Design review of the part built by this model. Coordinates are the model's own, in mm. A direction names the side the tool comes from. Coordinates: 2 decimals unless noted, no trailing zeros. Write each loop counter-clockwise with the first axis right and the second up, starting at its lowest first coordinate (ties: lowest second). Pieces come first, ordered by that corner, then holes.
Q1. The part is to be moulded in two halves that separate along Z. For faces 6 (the flat face through (-20, -57, 5)), 7 (the cylindrical face through (-15.33, -157.48, 58.78)), 8 (the conical face through (-43.789, -137.671, 58.425)), say which applies: released by +Z, released by -Z, zero draft, split by the parting line, or undercut.
Q2. Take a section at B-B, the plane z = 18.5. Write out the cut boundary in (x, y).
Q3. Take a section at A-A, the plane y = -15. Write out the cut boundary in (x, z).
Q4. For L1, parallel to Y at x = -15, z = 57; L2, parallel to Y at x = -45, z = 56.6; L3, parallel to X at y = -20, z = 48, list the stretches that pass through material, from the lowest coordinate up.
Q5. For pin 1 Ø6.5 at (x, y) = (-45, -155) entering from -Z; pin 2 Ø6 at (x, y) = (-15, -30) entering from +Z; pin 3 Ø1 at (x, z) = (-45.5, 35.5) entering from -Y, all flat-tipped, find the tip position at first contact; note any pin that passes through.
Q6. For faces 1 (the cylindrical face through (-16.75, -147.27, 2.46)), 2 (the cylindrical face through (-18.42, -162.483, 3.479)), 3 (the flat face through (-60, -79, 57)), 4 (the flat face through (-25, -160, 2)), 5 (the cylindrical face through (-42.69, -14.04, 58.78)), list the 3-axis set-ups (+Z, -Z, +X, -X, +Y, -Y) from which the entire face can be reached by the end or side of a thin tool; tool diameter is ignored.
from build123d import *

# Parameters (mm, degrees)
F0_R     = 2.5
F1_DEPTH = 5
F2_W     = 170
F2_H     = 50.3
F3_DEPTH = 5
F4_W     = 55
F4_H     = 50.3
F5_DEPTH = 5
F7_R     = 2.5
F8_DEPTH = 5
F9_SIZE  = 2
F10_SIZE = 2
F11_SIZE = 2
F12_R    = 2


# Not quite as in the source:
# - a feature names something its author has since deleted; it is built from what else it names


with BuildPart() as f1:
    # F0 (on Top) → F1 (new body)
    with BuildSketch(Plane.XY):
        with BuildLine():
            Line((-60, 0), (0, 0))
            Line((0, 0), (0, 150))
            Line((0, 150), (0, 170))
            Line((0, 170), (-15, 170))
            add(Edge.make_bspline(
                [(-15, 170), (-14.4841735922, 160.0600889734), (-13.9683471845, 150.1201779469), (-13.6234299021, 140.3529161241)],
                knots=[0, 0, 0, 0, 0.0906883322, 0.0906883322, 0.0906883322, 0.0906883322], degree=3))
            add(Edge.make_bspline(
                [(-13.6234299021, 140.3529161241), (-12.0632834056, 96.1731661082), (-14.5980537911, 42.9711861088), (-50.2193379026, 23.1925838291), (-60, 19.9139873857)],
                knots=[0.0906883322, 0.0906883322, 0.0906883322, 0.0906883322, 0.5008941728, 0.6275927921, 0.6275927921, 0.6275927921, 0.6275927921], degree=3))
            Line((-60, 19.9139873857), (-60, 0))
        make_face()
        with Locations((-21.5087961406, 26.8674660474)):
            Circle(F0_R, mode=Mode.SUBTRACT)
        with BuildLine():
            ThreePointArc((-23.6172004723, 150), (-16.6720280929, 147.1947606368), (-13.6234299021, 140.3529161241))
            add(Edge.make_bspline(
                [(-15, 170), (-14.4841735922, 160.0600889734), (-13.9683471845, 150.1201779469), (-13.6234299021, 140.3529161241)],
                knots=[0, 0, 0, 0, 0.0906883322, 0.0906883322, 0.0906883322, 0.0906883322], degree=3))
            Line((-15, 170), (-25, 170))
            Line((-25, 170), (-25, 150))
            Line((-25, 150), (-23.6172004723, 150))
        make_face()
        with Locations((-18.0946737528, 160.0040644407)):
            Circle(F0_R, mode=Mode.SUBTRACT)
    extrude(amount=F1_DEPTH)

    # F2 (on face) → F3 (join)
    with BuildSketch(Plane.YZ):
        with Locations((85, 30.15)):
            Rectangle(F2_W, F2_H)
    extrude(amount=-F3_DEPTH)

    # F4 (on face) → F5 (join)
    with BuildSketch(Plane.XZ):
        with Locations((-32.5, 30.15)):
            Rectangle(F4_W, F4_H)
    extrude(amount=-F5_DEPTH)

    # F7 (on face) → F8 (join)
    with BuildSketch(Plane.XY.offset(55.3)):
        Polygon((-15, 0), (0, 0), (0, 15), (0, 155), (0, 170), (-15, 170), (-45, 170), (-60, 170), (-60, 155), (-60, 15), (-60, 0), (-45, 0), align=None)
        with Locations((-45, 15)):
            Circle(F7_R, mode=Mode.SUBTRACT)
        with Locations((-45, 30)):
            Circle(F7_R, mode=Mode.SUBTRACT)
        with Locations((-15, 15)):
            Circle(F7_R, mode=Mode.SUBTRACT)
        with Locations((-15, 30)):
            Circle(F7_R, mode=Mode.SUBTRACT)
        with Locations((-45, 140)):
            Circle(F7_R, mode=Mode.SUBTRACT)
        with Locations((-45, 155)):
            Circle(F7_R, mode=Mode.SUBTRACT)
        with Locations((-15, 140)):
            Circle(F7_R, mode=Mode.SUBTRACT)
        with Locations((-15, 155)):
            Circle(F7_R, mode=Mode.SUBTRACT)
    extrude(amount=F8_DEPTH)

    # F9
    f9_edges = [f1.edges().sort_by_distance(p)[0] for p in [
        (-17.5, 140, 60.3),
        (-47.5, 140, 60.3),
        (-17.5, 30, 60.3),
        (-47.5, 30, 60.3),
    ]]
    chamfer(f9_edges, length=F9_SIZE)

    # F10
    f10_edges = [f1.edges().sort_by_distance(p)[0] for p in [
        (-47.5, 155, 55.3),
        (-17.5, 155, 55.3),
        (-47.5, 15, 55.3),
        (-17.5, 15, 55.3),
    ]]
    chamfer(f10_edges, length=F10_SIZE)

    # F11
    f11_edges = [f1.edges().sort_by_distance(p)[0] for p in [
        (-24.008796, 26.867466, 0),
        (-20.594674, 160.004064, 0),
    ]]
    chamfer(f11_edges, length=F11_SIZE)

    # F12
    f12_edges = [f1.edges().sort_by_distance(p)[0] for p in [
        (0, 0, 30.15),
        (-60, 0, 30.15),
        (-30, 0, 0),
        (0, 170, 30.15),
        (-60, 170, 57.8),
    ]]
    fillet(f12_edges, radius=F12_R)


with BuildPart() as f13_1:
    # F13: instance of F1
    add(f1.part.mirror(Plane(origin=(-30, 0, 31.15), x_dir=(1, 0, 0), z_dir=(0, -1, 0))))


solid = f13_1.part
Responses:
1. face 6: undercut
1. face 7: zero draft
1. face 8: released by +Z
2. outline: (-60, -5) - (-5, -5) - (-5, -170) - (-2, -170) arc R2 ccw to (0, -168) - (0, -2) arc R2 ccw to (-2, 0) - (-58, 0) arc R2 ccw to (-60, -2) - close
3. outline: (-60, 0) - (0, 0) - (0, 60.3) - (-12.5, 60.3) - (-12.5, 57.3) - (-10.5, 55.3) - (-5, 55.3) - (-5, 5) - (-60, 5) - close; (-60, 55.3) - (-49.5, 55.3) - (-47.5, 57.3) - (-47.5, 60.3) - (-60, 60.3) - close; (-42.5, 57.3) - (-40.5, 55.3) - (-19.5, 55.3) - (-17.5, 57.3) - (-17.5, 60.3) - (-42.5, 60.3) - close
4. L1: y = -170 to -157.8, -152.2 to -142.5, -137.5 to -32.5, -27.5 to -17.8, -12.2 to 0
4. L2: y = -170 to -158.2, -151.8 to -142.5, -137.5 to -32.5, -27.5 to -18.2, -11.8 to 0
4. L3: x = -5 to 0
5. pin 1: stops at z = 56.55
5. pin 2: stops at z = 58.8
5. pin 3: stops at y = -5
6. face 1: -Z, -X
6. face 2: -Z
6. face 3: +Z, -Z, -X, +Y, -Y
6. face 4: -Z, -X, -Y
6. face 5: +Z
